For this review, use the dimensioned drawing (mm, ordinates from the lowest corner) and the shaded views. Round coordinates to 2 decimals unless told otherwise and drop trailing zeros. Loops run counter-clockwise (first coordinate to the right, second up) from the corner with the lowest first, then second, coordinate; pieces in that order, holes last. Notation, with made-up numbers: (88.5, 53.25) - (134.5, 53.25) arc R26 ccw to (134.5, 86.25) - close; hole circle Ø4 at (71, 77.25). An arc over 180 degrees is marked (long way). Use one line per item in the form item = value. Start each with the question number.
(1) We need section D-D, the plane x = 45. Write out the cut boundary in (y, z).
(2) The part is to be moulded in two halves that separate along Z. For the marked faces 1, 2 and 3, say which applies: released by +Z, released by -Z, zero draft, split by the parting line, or undercut.
(3) We need section A-A, the plane x = 71. Write out the cut boundary in (y, z), then the cut area to 3 significant figures.
(4) We need section B-B, the plane z = 45. Write out the cut boundary in (x, y).
(5) We need section C-C, the plane y = 8.5. Write out the cut boundary in (x, z), then the cut area to 3 significant figures.
(6) For pin 1 (1 mm diameter, centred on x = 31, y = 3.5, fed in from -Z); pin 2 (4 mm diameter, centred on x = 48, z = 105, fed in from +Y); pin 3 (0.8 mm diameter, centred on x = 55, y = 3.5, fed in from +Z); pin 4 (3 mm diameter, centred on x = 45, y = 8.5, fed in from -Z), all flat-tipped, find the tip position at first contact; note any pin that passes through.
(7) Wall thickness on probe 1 along Y at (x, z) = (45, 1.2); probe 2 along X at (y, z) = (0.7, 45); probe 3 along Y at (x, z) = (8, 23): over which ranges is each line inside the solid? List them lowest first. Write a range as [from, to].
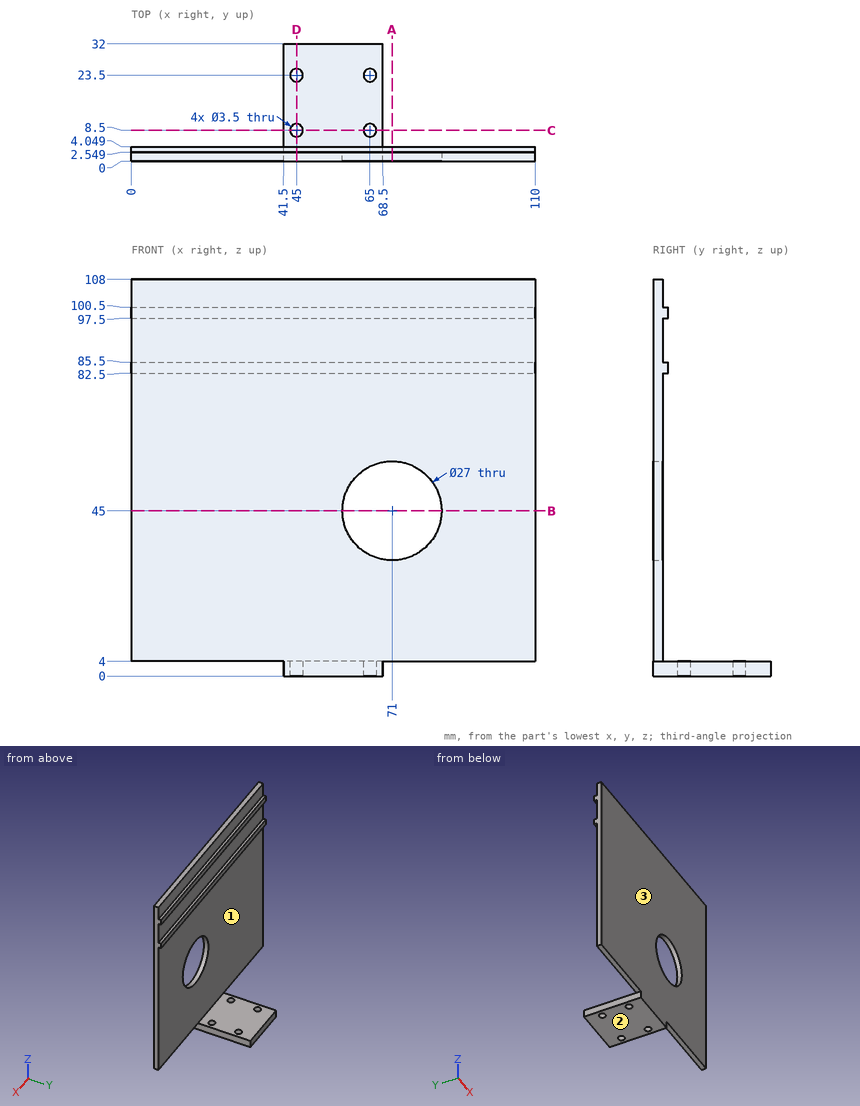
Data:
q1.outline = (0, 0) - (6.75, 0) - (6.75, 4) - (2.55, 4) - (2.55, 82.5) - (4.05, 82.5) - (4.05, 85.5) - (2.55, 85.5) - (2.55, 97.5) - (4.05, 97.5) - (4.05, 100.5) - (2.55, 100.5) - (2.55, 108) - (0, 108) - close; (10.25, 0) - (21.75, 0) - (21.75, 4) - (10.25, 4) - close; (25.25, 0) - (32, 0) - (32, 4) - (25.25, 4) - close
q2.face_1 = undercut
q2.face_2 = released by -Z
q2.face_3 = zero draft
q3.outline = (0, 4) - (2.55, 4) - (2.55, 31.5) - (0, 31.5) - close; (0, 58.5) - (2.55, 58.5) - (2.55, 82.5) - (4.05, 82.5) - (4.05, 85.5) - (2.55, 85.5) - (2.55, 97.5) - (4.05, 97.5) - (4.05, 100.5) - (2.55, 100.5) - (2.55, 108) - (0, 108) - close
q3.area = 205 mm^2
q4.outline = (0, 0) - (57.5, 0) - (57.5, 2.55) - (0, 2.55) - close; (84.5, 0) - (110, 0) - (110, 2.55) - (84.5, 2.55) - close
q5.outline = (41.5, 0) - (43.25, 0) - (43.25, 4) - (41.5, 4) - close; (46.75, 0) - (63.25, 0) - (63.25, 4) - (46.75, 4) - close; (66.75, 0) - (68.5, 0) - (68.5, 4) - (66.75, 4) - close
q5.area = 80.0 mm^2
q6.pin_1 = 82.5
q6.pin_2 = 2.55
q6.pin_3 = 100.5
q6.pin_4 = through
q7.probe_1 = [0, 6.75], [10.25, 21.75], [25.25, 32]
q7.probe_2 = [0, 57.5], [84.5, 110]
q7.probe_3 = [0, 2.55]
